Could you check a few things on this drawing? It's one solid part, dimensions in mm from its lowest x, y, z. A direction names the side the tool comes from. Coordinates: 2 decimals unless noted, no trailing zeros. Write each loop counter-clockwise with the first axis right and the second up, starting at its lowest first coordinate (ties: lowest second). Pieces come first, ordered by that corner, then holes. Notation, with made-up numbers: M -22.5,73.5 L 23.5,73.5 A25 cw 23.5,104.5 Z; hole C 61.25,44 d7. An arc over 180 degrees is marked long. Use a Markdown table: item, result.
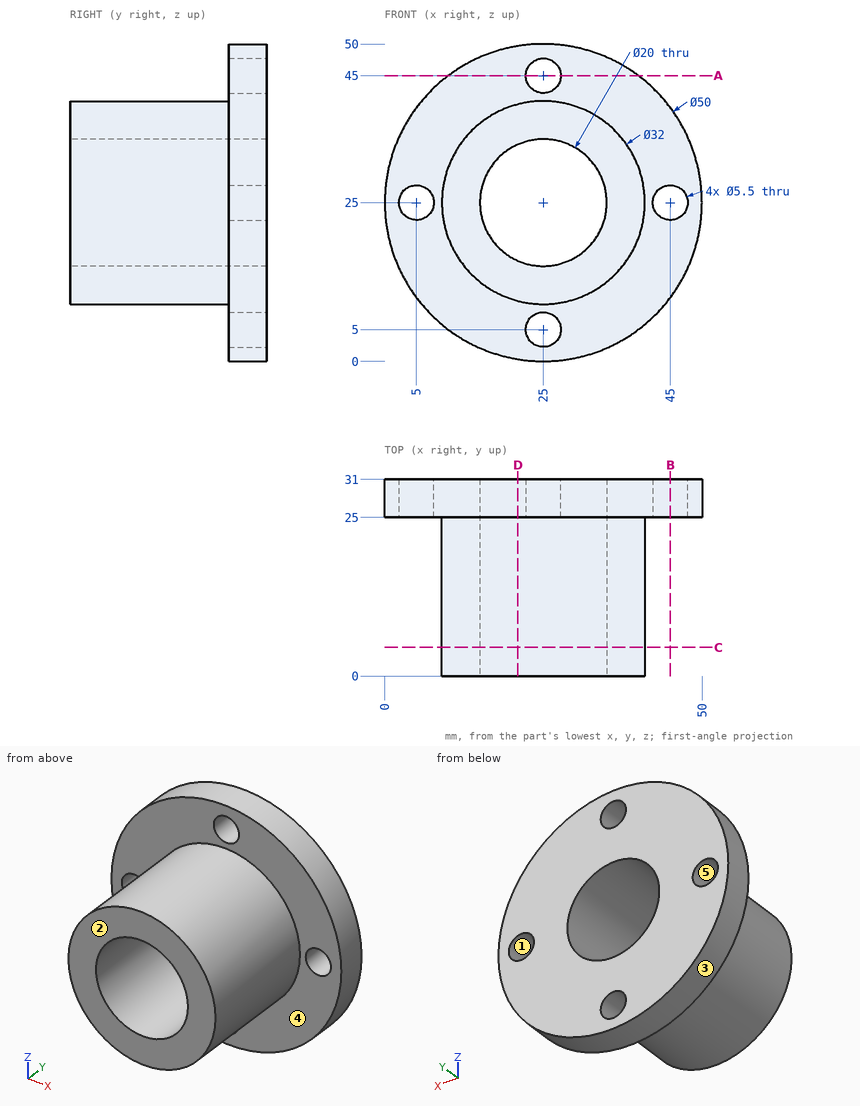
1. Which directions (+Z, -Z, +X, -X, +Y, -Y) give clear straight access to the entire face, cutting with the end or side of a thin tool? Please do the marked faces 4 and 5.
Answers follow:
| item | result |
|---|---|
| face 4 | -Y |
| face 5 | +Y, -Y |
2. Suppose I cut it at C-C on y = 4.5. Write out the boundary of the cut face in (x, z).
Answers follow:
| item | result |
|---|---|
| outline | C 25,25 d32; hole C 25,25 d20 |
3. We'd pull the mould along X, two halves only. Please class the marked faces 1, 2 and 3: +X half, -X half, draft (parallel to the pull), parting line (faces both ways), or undercut.
Answers follow:
| item | result |
|---|---|
| face 1 | undercut |
| face 2 | draft |
| face 3 | parting line |
4. I need wall thicknesses on probe 1 along Y at (x, z) = (10.5, 15.5); probe 2 along X at (y, z) = (25.5, 29); probe 3 along Z at (x, y) = (26, 10). Which ranges of each line are inside material? Lowest first, please.
Answers follow:
| item | result |
|---|---|
| probe 1 | y = 25 to 31 |
| probe 2 | x = 0.32 to 15.83, 34.17 to 49.68 |
| probe 3 | z = 9.03 to 15.05, 34.95 to 40.97 |
5. Will these pins go through, and if not, where does the flat tip stop? pin 1 Ø3 at (y, z) = (20, 24) entering from -X; pin 2 Ø8 at (x, y) = (26.5, 12.5) entering from -Z; pin 3 Ø2 at (y, z) = (4.5, 28) entering from +X.
Answers follow:
| item | result |
|---|---|
| pin 1 | stops at x = 9 |
| pin 2 | stops at z = 9 |
| pin 3 | stops at x = 40.87 |
6. Suppose I cut it at B-B on x = 45. Write out the boundary of the cut face in (y, z), and give its area (3 significant figures).
Answers follow:
| item | result |
|---|---|
| outline | M 25,10 L 31,10 L 31,22.25 L 25,22.25 Z; M 25,27.75 L 31,27.75 L 31,40 L 25,40 Z |
| area | 147 mm2 |
7. Suppose I cut it at A-A on z = 45. Write out the boundary of the cut face in (x, y).
Answers follow:
| item | result |
|---|---|
| outline | M 10,25 L 22.25,25 L 22.25,31 L 10,31 Z; M 27.75,25 L 40,25 L 40,31 L 27.75,31 Z |
8. Suppose I cut it at D-D on x = 21. Write out the boundary of the cut face in (y, z), and give its area (3 significant figures).
Answers follow:
| item | result |
|---|---|
| outline | M 0,9.51 L 25,9.51 L 25,0.32 L 31,0.32 L 31,15.83 L 0,15.83 Z; M 0,34.17 L 31,34.17 L 31,49.68 L 25,49.68 L 25,40.49 L 0,40.49 Z |
| area | 502 mm2 |
